The model under review builds one solid part; all positions refer to its coordinate system, in mm. A direction names the side the tool comes from. Coordinates: 2 decimals unless noted, no trailing zeros. Loops run counter-clockwise (first coordinate to the right, second up) from the corner with the lowest first, then second, coordinate; pieces in that order, holes last. Notation, with made-up numbers: (-10.5, 55) - (9.5, 55) arc R29 cw to (9.5, 88) - close; hole circle Ø11 at (-3, 35). An arc over 180 degrees is marked (long way). Answer in a Markdown table with one row per item. Add a question column.
(1) We need section B-B on y = -1.5. Write out the cut boundary in (x, z).
(2) We need section C-C on y = 26. Write out the cut boundary in (x, z), plus the area to 3 significant figures.
(3) Mouldability with a two-part tool opening along X and no side actions: class faces 1 (the flat face through (-7, 29, 3.81)), 2 (the flat face through (7, 0, 6.35)) as +X half, -X half, draft (parallel to the pull), parting line (faces both ways), or undercut.
(4) For line 1 along X through (y, z) = (0, 5.7); line 2 along X through (y, z) = (-1, 3), list the stretches that pass through material, from the lowest coordinate up.
(5) We need section A-A on x = -1. Write out the cut boundary in (y, z) (3 decimals).
(6) We need section D-D on y = 11. Write out the cut boundary in (x, z).
(7) Machinability: for faces 3 (the flat face through (0, -30, 3.81)), 4 (the cylindrical face through (3.32, 1.04, 5.71)), 5 (the cylindrical face through (26.578, -8.551, 1.878)), which of the approach directions +Z, -Z, +X, -X, +Y, -Y give a long, thin tool a straight path to every point of the face, cutting with its end or side? Answer none if there is none.
(8) For P1, Ø3, axis at x = 24, y = -21.5, coming from the -Z side; P2, Ø3, axis at x = 25, z = 3, coming from the -Y side; P3, Ø2, axis at y = -9, z = 5, coming from the -X side, all flat-tipped, find the tip position at first contact; note any pin that passes through.
from build123d import *

# Parameters (mm, degrees)
F0_R     = 31.728285
F0_R_2   = 3.478838
F1_DEPTH = 6.35
F3_DEPTH = 5.08
F4_R     = 3.81
F5_DEPTH = 3.81


with BuildPart() as f1:
    # F0 (on Top) → F1 (new body)
    with BuildSketch(Plane.XY):
        Circle(F0_R)
        Circle(F0_R_2, mode=Mode.SUBTRACT)
    extrude(amount=F1_DEPTH)

    # F2 (on Top) → F3 (cut)
    with BuildSketch(Plane.XY):
        Polygon((6.35, -3.666174), (6.35, 3.666174), (0, 7.332348), (-6.35, 3.666174), (-6.35, -3.666174), (0, -7.332348), align=None)
    extrude(amount=F3_DEPTH, mode=Mode.SUBTRACT)

    # F4 (on Top) → F5 (cut)
    with BuildSketch(Plane.XY):
        with Locations((0, -31.728285)):
            Circle(F4_R)
        with Locations((12.905056, -28.98523)):
            Circle(F4_R)
        with Locations((23.578711, -21.230366)):
            Circle(F4_R)
        with Locations((30.175392, -9.804579)):
            Circle(F4_R)
        with Locations((31.554474, 3.316509)):
            Circle(F4_R)
        with Locations((27.477501, 15.864142)):
            Circle(F4_R)
        with Locations((18.649418, 25.668721)):
            Circle(F4_R)
        with Locations((6.596681, 31.034946)):
            Circle(F4_R)
        with Locations((-6.596681, 31.034946)):
            Circle(F4_R)
        with Locations((-18.649418, 25.668721)):
            Circle(F4_R)
        with Locations((-27.477501, 15.864142)):
            Circle(F4_R)
        with Locations((-31.554474, 3.316509)):
            Circle(F4_R)
        with Locations((-30.175392, -9.804579)):
            Circle(F4_R)
        with Locations((-23.578711, -21.230366)):
            Circle(F4_R)
        with Locations((-12.905056, -28.98523)):
            Circle(F4_R)
    extrude(amount=F5_DEPTH, mode=Mode.SUBTRACT)


solid = f1.part
Outcome:
| question | item | result |
|---|---|---|
| 1 | outline | (-31.69, 0) - (-6.35, 0) - (-6.35, 5.08) - (-3.14, 5.08) - (-3.14, 6.35) - (-31.69, 6.35) - close; (3.14, 5.08) - (6.35, 5.08) - (6.35, 0) - (31.69, 0) - (31.69, 6.35) - (3.14, 6.35) - close |
| 2 | outline | (-18.18, 3.81) - (-14.85, 3.81) - (-14.85, 0) - (14.85, 0) - (14.85, 3.81) - (18.18, 3.81) - (18.18, 6.35) - (-18.18, 6.35) - close |
| 2 | area | 206 mm² |
| 3 | face 1 | undercut |
| 3 | face 2 | draft |
| 4 | line 1 | -31.73 to -3.48, 3.48 to 31.73 |
| 4 | line 2 | -31.71 to -6.35, 6.35 to 31.71 |
| 5 | outline | (-31.713, 3.81) - (-28.052, 3.81) - (-28.052, 0) - (-6.755, 0) - (-6.755, 5.08) - (-3.332, 5.08) - (-3.332, 6.35) - (-31.713, 6.35) - close; (3.332, 5.08) - (6.755, 5.08) - (6.755, 0) - (31.713, 0) - (31.713, 6.35) - (3.332, 6.35) - close |
| 6 | outline | (-29.76, 0) - (29.76, 0) - (29.76, 6.35) - (-29.76, 6.35) - close |
| 7 | face 3 | -Z, -Y |
| 7 | face 4 | +Z, -Z |
| 7 | face 5 | -Z |
| 8 | P1 | z = 3.81 |
| 8 | P2 | y = -21.05 |
| 8 | P3 | x = -30.7 |
